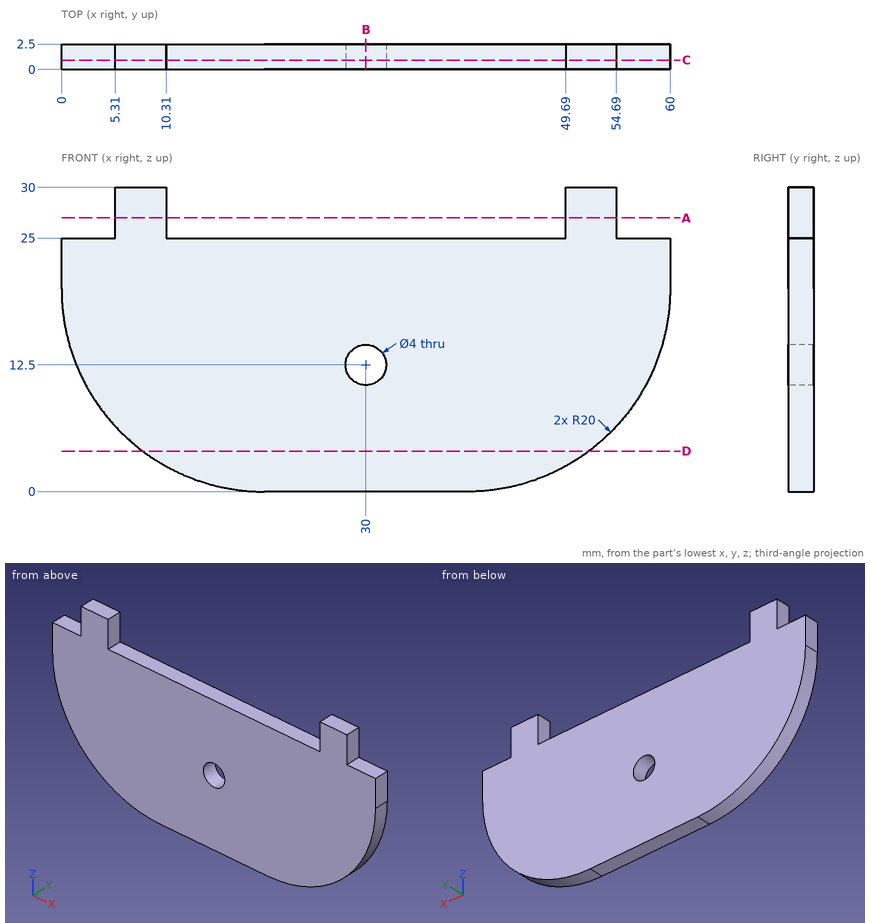
Geometry: see drawing. Coordinates: mm, zero at the bounding-box minimum. Give positions to 0.01 mm unless a question says otherwise; leave off trailing zeros. Order: outer loops, then holes, each group sorted by start corner. A loop starts at its lowest first (then second) coordinate and runs counter-clockwise, first axis right, second up. Notation, with made-up numbers: (39, 53.5) -> (72, 53.5) arc R20 ccw to (72, 81.5) -> close; hole circle Ø1 at (-28, 66). An arc over 180 degrees is marked (long way). Write item = value, one per line.
Q1. Cut plane A-A, the plane z = 27. Output: boundary loops of the cut face in (x, y), and give its area (3 significant figures).
Data:
outline = (5.31, 0) -> (10.31, 0) -> (10.31, 2.5) -> (5.31, 2.5) -> close; (49.69, 0) -> (54.69, 0) -> (54.69, 2.5) -> (49.69, 2.5) -> close
area = 25.0 mm^2
Q2. Pin query (flat end, axial travel): pin 1 (0.8 mm diameter, centred on y = 0.5, z = 28, fed in from -X); pin 2 (1.2 mm diameter, centred on x = 22.5, y = 1, fed in from +Z). Return the tip coordinate at first contact, or that it passes through.
Data:
pin_1 = 5.31
pin_2 = 25
Q3. Cut plane B-B, the plane x = 30. Output: boundary loops of the cut face in (y, z).
Data:
outline = (0, 0) -> (2.5, 0) -> (2.5, 10.5) -> (0, 10.5) -> close; (0, 14.5) -> (2.5, 14.5) -> (2.5, 25) -> (0, 25) -> close
Q4. Cut plane C-C, the plane y = 0.9. Output: boundary loops of the cut face in (x, z).
Data:
outline = (0, 20) arc R20 ccw to (20, 0) -> (40, 0) arc R20 ccw to (60, 20) -> (60, 25) -> (54.69, 25) -> (54.69, 30) -> (49.69, 30) -> (49.69, 25) -> (10.31, 25) -> (10.31, 30) -> (5.31, 30) -> (5.31, 25) -> (0, 25) -> close; hole circle Ø4 at (30, 12.5)
Q5. Material intervals for line 1 (X direction, y = 2.4, z = 26); line 2 (Z direction, x = 24, y = 1.4); line 3 (X direction, y = 1.1, z = 12.5), sorted ascending. Write a range as from..to.
Data:
line_1 = 5.31..10.31, 49.69..54.69
line_2 = 0..25
line_3 = 1.46..28, 32..58.54
Q6. Cut plane D-D, the plane z = 4. Output: boundary loops of the cut face in (x, y), and give its area (3 significant figures).
Data:
outline = (8, 0) -> (52, 0) -> (52, 2.5) -> (8, 2.5) -> close
area = 110 mm^2
